Verification items for the finished model (mm, model axes). Give positions to 0.01 mm unless a question says otherwise; leave off trailing zeros. Order: outer loops, then holes, each group sorted by start corner. A loop starts at its lowest first (then second) coordinate and runs counter-clockwise, first axis right, second up.
(1) Scan lines: L1, parallel to X at y = 0, z = 7.75; L2, parallel to Z at x = -1, y = -14.5. Record each from-to range of solid material in increasing order.
(2) Gauge pin test, flat end, axial feed: pin 1 (5.5 mm diameter, centred on x = 0, y = 0, fed in from +Z). Record the tip position at first contact, or that the pin passes through.
(3) Sectioned sample at C-C on y = 11.31. Record the cut outline in (x, z), plus the area to 3 significant figures.
(4) Sectioned sample at B-B on z = 4. Count the separate pieces of the cut face and the enclosed holes in it, plus the area to 3 significant figures.
(5) Sectioned sample at A-A on y = 0. Record the cut outline in (x, z).
```python
from build123d import *

# Parameters (mm, degrees)
SKETCH1_W           = 40
SKETCH1_H           = 40
BOSS_EXTRUDE1_DEPTH = 11
CUT_EXTRUDE1_DEPTH  = 47.054315759
SKETCH4_R           = 2
SKETCH4_R_2         = 3
CUT_EXTRUDE2_DEPTH  = 31.347981811


with BuildPart() as part:
    # Sketch1 → Boss-Extrude1 (new body)
    with BuildSketch(Plane.XY):
        Rectangle(SKETCH1_W, SKETCH1_H)
    extrude(amount=BOSS_EXTRUDE1_DEPTH)

    # Sketch3 → Cut-Extrude1 (cut, through all)
    with BuildSketch(Plane(origin=(20, 0, 0), x_dir=(0, 0, -1), z_dir=(1, 0, 0))):
        with BuildLine():
            Line((-11, -18.769), (-11, -16.769))
            Line((-11, -16.769), (-2.8, -16.769))
            ThreePointArc((-2.8, -16.769), (-1.8, -17.769), (-2.8, -18.769))
            Line((-2.8, -18.769), (-11, -18.769))
        make_face()
        with BuildLine():
            Line((-2.8, -13.538), (-11, -13.538))
            Line((-11, -13.538), (-11, -15.538))
            Line((-11, -15.538), (-2.8, -15.538))
            ThreePointArc((-2.8, -15.538), (-1.8, -14.538), (-2.8, -13.538))
        make_face()
        with BuildLine():
            Line((-2.8, -10.307), (-11, -10.307))
            Line((-11, -10.307), (-11, -12.307))
            Line((-11, -12.307), (-2.8, -12.307))
            ThreePointArc((-2.8, -12.307), (-1.8, -11.307), (-2.8, -10.307))
        make_face()
        with BuildLine():
            Line((-2.8, -7.076), (-11, -7.076))
            Line((-11, -7.076), (-11, -9.076))
            Line((-11, -9.076), (-2.8, -9.076))
            ThreePointArc((-2.8, -9.076), (-1.8, -8.076), (-2.8, -7.076))
        make_face()
        with BuildLine():
            Line((-2.8, -3.845), (-11, -3.845))
            Line((-11, -3.845), (-11, -5.845))
            Line((-11, -5.845), (-2.8, -5.845))
            ThreePointArc((-2.8, -5.845), (-1.8, -4.845), (-2.8, -3.845))
        make_face()
        with BuildLine():
            Line((-2.8, -0.614), (-11, -0.614))
            Line((-11, -0.614), (-11, -2.614))
            Line((-11, -2.614), (-2.8, -2.614))
            ThreePointArc((-2.8, -2.614), (-1.8, -1.614), (-2.8, -0.614))
        make_face()
        with BuildLine():
            Line((-2.8, 2.617), (-11, 2.617))
            Line((-11, 2.617), (-11, 0.617))
            Line((-11, 0.617), (-2.8, 0.617))
            ThreePointArc((-2.8, 0.617), (-1.8, 1.617), (-2.8, 2.617))
        make_face()
        with BuildLine():
            Line((-2.8, 5.848), (-11, 5.848))
            Line((-11, 5.848), (-11, 3.848))
            Line((-11, 3.848), (-2.8, 3.848))
            ThreePointArc((-2.8, 3.848), (-1.8, 4.848), (-2.8, 5.848))
        make_face()
        with BuildLine():
            Line((-2.8, 9.079), (-11, 9.079))
            Line((-11, 9.079), (-11, 7.079))
            Line((-11, 7.079), (-2.8, 7.079))
            ThreePointArc((-2.8, 7.079), (-1.8, 8.079), (-2.8, 9.079))
        make_face()
        with BuildLine():
            Line((-2.8, 12.31), (-11, 12.31))
            Line((-11, 12.31), (-11, 10.31))
            Line((-11, 10.31), (-2.8, 10.31))
            ThreePointArc((-2.8, 10.31), (-1.8, 11.31), (-2.8, 12.31))
        make_face()
        with BuildLine():
            Line((-2.8, 15.541), (-11, 15.541))
            Line((-11, 15.541), (-11, 13.541))
            Line((-11, 13.541), (-2.8, 13.541))
            ThreePointArc((-2.8, 13.541), (-1.8, 14.541), (-2.8, 15.541))
        make_face()
        with BuildLine():
            Line((-2.8, 18.772), (-11, 18.772))
            Line((-11, 18.772), (-11, 16.772))
            Line((-11, 16.772), (-2.8, 16.772))
            ThreePointArc((-2.8, 16.772), (-1.8, 17.772), (-2.8, 18.772))
        make_face()
    extrude(amount=-CUT_EXTRUDE1_DEPTH, mode=Mode.SUBTRACT)

    # Sketch4 → Cut-Extrude2 (cut, through all)
    with BuildSketch(Plane(origin=(0, 0, 0), x_dir=(-1, 0, 0), z_dir=(0, 0, -1))):
        with Locations((16, -15.5)):
            Circle(SKETCH4_R)
        with Locations((-16, -15.5)):
            Circle(SKETCH4_R)
        Circle(SKETCH4_R_2)
    extrude(amount=-CUT_EXTRUDE2_DEPTH, mode=Mode.SUBTRACT)


solid = part.part
```
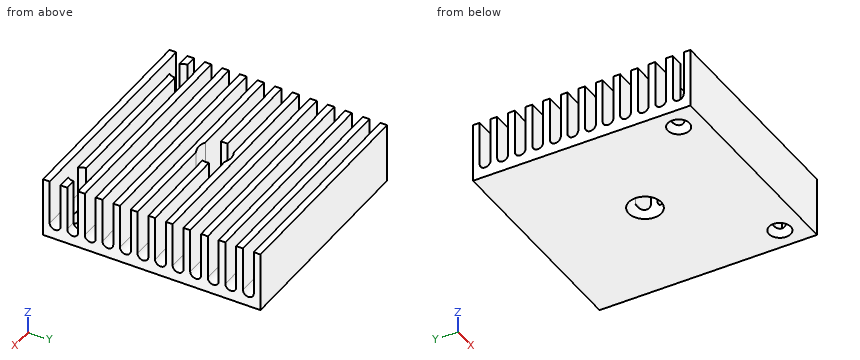
Ans:
1. L1: x = -20 to -3, 3 to 20
1. L2: z = 0 to 1.8
2. pin 1: passes through
3. outline: (-20, 0) - (20, 0) - (20, 1.8) - (-20, 1.8) - close
3. area: 72.0 mm2
4. separate pieces: 16
4. enclosed holes: 0
4. area: 622 mm2
5. outline: (-20, 0) - (-3, 0) - (-3, 11) - (-20, 11) - close; (3, 0) - (20, 0) - (20, 11) - (3, 11) - close
